Here's how the part is built. I have some questions about the finished solid (model axes, mm). Face numbers are marked on the shaded views. Coordinates: 2 decimals unless noted, no trailing zeros. Loops run counter-clockwise (first coordinate to the right, second up) from the corner with the lowest first, then second, coordinate; pieces in that order, holes last. Notation, with made-up numbers: (76, 87) -> (118, 87) arc R30 cw to (118, 111) -> close; hole circle Ø6 at (89.25, -24). An arc over 180 degrees is marked (long way). Answer as a JSON object with one key per item and string values. Group by question number.
Q1. I want a section at B-B on x = 0. Write out the boundary of the cut face in (y, z).
Q2. I want a section at A-A on z = 0. Write out the boundary of the cut face in (x, y).
Q3. I need wall thicknesses on line 1 (Z direction, x = 0, y = 29); line 2 (Z direction, x = 4.5, y = 93); line 3 (X direction, y = 37, z = -3.5). Which ranges of each line are inside material? Lowest first, please.
Q4. I'm going to push flat-ended pins straight in: pin 1 (12 mm diameter, centred on y = 36.5, z = 34, fed in from +X); pin 2 (4 mm diameter, centred on x = -20, y = 155.5, fed in from +Z); pin 3 (2 mm diameter, centred on y = 76, z = 20.5, fed in from -X); pin 4 (8 mm diameter, centred on y = 7.5, z = 0, fed in from -X). Where does each tip first touch, or does it pass through?
Q5. I want a section at D-D on z = 33. Write out the boundary of the cut face in (x, y), then the cut area to 3 significant figures.
Q6. Thinking about a two-plate mould opening in Z: for the marked faces 1 and 2, which applies, released by +Z, released by -Z, zero draft, split by the parting line, or undercut?
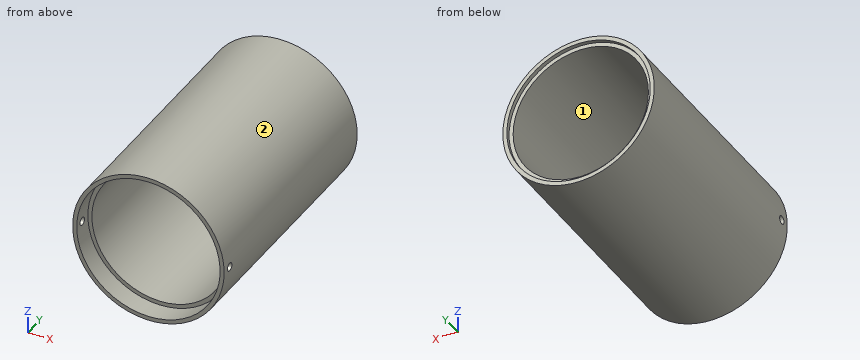
```python
from build123d import *

# Parameters (mm, degrees)
SKETCH1_R               = 56
SKETCH1_R_2             = 50
EXTRUDE_THIN1_DEPTH     = 180
SKETCH2_R               = 53
CUT_EXTRUDE1_DEPTH      = 3
CUT_EXTRUDE2_START      = -15
SKETCH3_R               = 53
CUT_EXTRUDE2_DEPTH      = 15
CUT_EXTRUDE3_DEPTH      = 218.754448864
CUT_EXTRUDE3_DEPTH_BACK = 218.754448864
SKETCH5_R               = 3


with BuildPart() as part:
    # Sketch1 → Extrude-Thin1 (new body)
    with BuildSketch(Plane(origin=(0, 0, 0), x_dir=(1, 0, 0), z_dir=(0, 1, 0))):
        Circle(SKETCH1_R)
        Circle(SKETCH1_R_2, mode=Mode.SUBTRACT)
    extrude(amount=EXTRUDE_THIN1_DEPTH)

    # Sketch2 → Cut-Extrude1 (cut)
    with BuildSketch(Plane(origin=(0, 180, 0), x_dir=(1, 0, 0), z_dir=(0, 1, 0))):
        with Locations(Location((0, 0, 0), (0, 0, 270))):
            Circle(SKETCH2_R)
    extrude(amount=-CUT_EXTRUDE1_DEPTH, mode=Mode.SUBTRACT)

    # Sketch3 → Cut-Extrude2 (cut)
    with BuildSketch(Plane.XZ.offset(CUT_EXTRUDE2_START)):
        with Locations(Location((0, 0, 0), (0, 0, 90))):
            Circle(SKETCH3_R)
    extrude(amount=CUT_EXTRUDE2_DEPTH, mode=Mode.SUBTRACT)

    # Sketch5 → Cut-Extrude3 (cut, two sides: drawn at the far end of the back side and taken through both)
    with BuildSketch(Plane.ZY.offset(-53).offset(-CUT_EXTRUDE3_DEPTH_BACK)):
        with Locations(Location((0, 7.5, 0), (0, 0, 180))):
            Circle(SKETCH5_R)
    extrude(amount=CUT_EXTRUDE3_DEPTH + CUT_EXTRUDE3_DEPTH_BACK, mode=Mode.SUBTRACT)


solid = part.part
```
Result set:
{
 "1": {"outline": "(0, -56) -> (180, -56) -> (180, -53) -> (177, -53) -> (177, -50) -> (15, -50) -> (15, -53) -> (0, -53) -> close; (0, 53) -> (15, 53) -> (15, 50) -> (177, 50) -> (177, 53) -> (180, 53) -> (180, 56) -> (0, 56) -> close"},
 "2": {"outline": "(-56, 0) -> (-53, 0) -> (-53, 4.5) -> (-56, 4.5) -> close; (-56, 10.5) -> (-53, 10.5) -> (-53, 15) -> (-50, 15) -> (-50, 177) -> (-53, 177) -> (-53, 180) -> (-56, 180) -> close; (50, 15) -> (53, 15) -> (53, 10.5) -> (56, 10.5) -> (56, 180) -> (53, 180) -> (53, 177) -> (50, 177) -> close; (53, 0) -> (56, 0) -> (56, 4.5) -> (53, 4.5) -> close"},
 "3": {"line 1": "z = -56 to -50, 50 to 56", "line 2": "z = -55.82 to -49.8, 49.8 to 55.82", "line 3": "x = -55.89 to -49.88, 49.88 to 55.89"},
 "4": {"pin 1": "stops at x = 48.5", "pin 2": "stops at z = 53.03", "pin 3": "stops at x = -52.5", "pin 4": "stops at x = -56"},
 "5": {"outline": "(-45.24, 0) -> (-41.47, 0) -> (-41.47, 15) -> (-37.56, 15) -> (-37.56, 177) -> (-41.47, 177) -> (-41.47, 180) -> (-45.24, 180) -> close; (37.56, 15) -> (41.47, 15) -> (41.47, 0) -> (45.24, 0) -> (45.24, 180) -> (41.47, 180) -> (41.47, 177) -> (37.56, 177) -> close", "area": "2,620 mm²"},
 "6": {"face 1": "undercut", "face 2": "split by the parting line"}
}
